from build123d import *

# Parameters (mm, degrees)
F1_DEPTH = 8.1
F3_DEPTH = 0.7
F5_DEPTH = 4.1
F6_DEPTH = 2.7


with BuildPart() as f1:
    # F0 (on Top) → F1 (new body)
    with BuildSketch(Plane.XY):
        Polygon((-9.85, -9.65), (9.85, -9.65), (9.85, 5.25), (13.5, 5.25), (13.5, 5.95), (9.85, 5.95), (9.85, 9.65), (-9.85, 9.65), (-9.85, 5.95), (-13.5, 5.95), (-13.5, 5.25), (-9.85, 5.25), align=None)
    extrude(amount=F1_DEPTH)

    # F2 (on face) → F3 (cut, through all)
    with BuildSketch(Plane(origin=(0, 5.95, 0), x_dir=(-1, 0, 0), z_dir=(0, 1, 0))):
        with BuildLine():
            ThreePointArc((-11.65, 0), (-13.015604, 1.823736), (-13.5, 4.05))
            Line((-13.5, 4.05), (-13.5, 0))
            Line((-13.5, 0), (-11.65, 0))
        make_face()
        with BuildLine():
            ThreePointArc((-13.5, 4.05), (-13.015604, 6.276264), (-11.65, 8.1))
            Line((-11.65, 8.1), (-13.5, 8.1))
            Line((-13.5, 8.1), (-13.5, 4.05))
        make_face()
        with BuildLine():
            Line((13.5, 8.1), (11.65, 8.1))
            ThreePointArc((11.65, 8.1), (13.015604, 6.276264), (13.5, 4.05))
            Line((13.5, 4.05), (13.5, 8.1))
        make_face()
        with BuildLine():
            Line((13.5, 0), (13.5, 4.05))
            ThreePointArc((13.5, 4.05), (13.015604, 1.823736), (11.65, 0))
            Line((11.65, 0), (13.5, 0))
        make_face()
    extrude(amount=-F3_DEPTH, mode=Mode.SUBTRACT)

    # F4 (on face) → F5 (join)
    with BuildSketch(Plane(origin=(0, 9.65, 0), x_dir=(-1, 0, 0), z_dir=(0, 1, 0))):
        with BuildLine():
            ThreePointArc((5.8, 8.1), (3.82183, 7.584027), (2.347701, 6.167577))
            ThreePointArc((2.347701, 6.167577), (1.75, 4.05), (2.347701, 1.932423))
            ThreePointArc((2.347701, 1.932423), (3.82183, 0.515973), (5.8, 0))
            ThreePointArc((5.8, 0), (8.663782, 1.186218), (9.85, 4.05))
            ThreePointArc((9.85, 4.05), (8.663782, 6.913782), (5.8, 8.1))
        make_face()
    extrude(amount=F5_DEPTH)

    # F4 (on face) → F6 (join)
    with BuildSketch(Plane(origin=(0, 9.65, 0), x_dir=(-1, 0, 0), z_dir=(0, 1, 0))):
        with BuildLine():
            ThreePointArc((2.347701, 1.932423), (1.75, 4.05), (2.347701, 6.167577))
            ThreePointArc((2.347701, 6.167577), (-0.85, 4.05), (2.347701, 1.932423))
        make_face()
    extrude(amount=F6_DEPTH)


solid = f1.part
For this review, take the finished solid that the model builds, in its own axes (mm). A direction names the side the tool comes from. Round coordinates to 2 decimals unless told otherwise and drop trailing zeros. Order: outer loops, then holes, each group sorted by start corner. A loop starts at its lowest first (then second) coordinate and runs counter-clockwise, first axis right, second up. Notation, with made-up numbers: M -29.5,42.25 L 12.5,42.25 A13 ccw 12.5,67.25 Z; hole C 87.25,-33.5 d1. An arc over 180 degrees is marked long. Use a Markdown table: item, result. Add a question column.
Item 1: Insertion check: pin 1 (4 mm diameter, centred on y = 8, z = 4.5, fed in from -X); pin 2 (2.5 mm diameter, centred on x = 0, z = 3, fed in from +Y); pin 3 (1.8 mm diameter, centred on x = 11, z = 4, fed in from -Y). Each pin has a flat end and moves straight along its axis. Give the tip position at first contact, or say it passes through.
Item 2: Add section C-C, the plane z = 5. Give the boundary of the cut face in (x, y).
Item 3: To check wall thickness, follow line 1 along X through (y, z) = (1.5, 6.75); line 2 along Y through (x, z) = (3.25, 6.25); line 3 along Y through (x, z) = (-12, 6.75). State the ranges of each line that lie inside material, in increasing order.
Item 4: Tool access review of faces 1 (the flat face through (11, 5.25, 4)), 2 (the flat face through (-9, 9.65, 7)), 3 (the flat face through (9.85, 8, 4)), 4 (the flat face through (-11, 5.25, 4)): name each direction out of +Z, -Z, +X, -X, +Y, -Y from which nothing blocks a thin tool from reaching the whole face with its end or side.
Item 5: Add section D-D, the plane y = -5.75. Give the boundary of the cut face in (x, z), then the cut area to 3 significant figures.
Item 6: Add section B-B, the plane y = 11.25. Give the boundary of the cut face in (x, z), then the cut area to 3 significant figures.
Item 7: Add section A-A, the plane x = -1.45. Give the boundary of the cut face in (y, z).
Item 8: Mouldability with a two-part tool opening along X and no side actions: class faces 5 (the cylindrical face through (0.85, 10.98, 4.11)), 6 (the flat face through (9.85, -2, 4)), 7 (the flat face through (-11, 5.95, 4)) as released by +X, released by -X, zero draft, split by the parting line, or undercut.
Geometry results:
| question | item | result |
|---|---|---|
| 1 | pin 1 | stops at x = -9.85 |
| 1 | pin 2 | stops at y = 12.35 |
| 1 | pin 3 | stops at y = 5.25 |
| 2 | outline | M -13.42,5.25 L -9.85,5.25 L -9.85,-9.65 L 9.85,-9.65 L 9.85,5.25 L 13.42,5.25 L 13.42,5.95 L 9.85,5.95 L 9.85,9.65 L 0.64,9.65 L 0.64,12.35 L -1.86,12.35 L -1.86,13.75 L -9.74,13.75 L -9.74,9.65 L -9.85,9.65 L -9.85,5.95 L -13.42,5.95 Z |
| 3 | line 1 | x = -9.85 to 9.85 |
| 3 | line 2 | y = -9.65 to 9.65 |
| 3 | line 3 | y = 5.25 to 5.95 |
| 4 | face 1 | +Z, -Z, +X, -Y |
| 4 | face 2 | +Z, -X, +Y |
| 4 | face 3 | +Z, -Z, +X, +Y |
| 4 | face 4 | +Z, -Z, -X, -Y |
| 5 | outline | M -9.85,0 L 9.85,0 L 9.85,8.1 L -9.85,8.1 Z |
| 5 | area | 160 mm² |
| 6 | outline | M -9.85,4.05 A4.05 ccw -5.8,0 A4.05 ccw -2.35,1.93 A2.3 ccw long -2.35,6.17 A4.05 ccw -5.8,8.1 A4.05 ccw Z |
| 6 | area | 62.1 mm² |
| 7 | outline | M -9.65,0 L 9.65,0 L 9.65,1.75 L 12.35,1.75 L 12.35,6.35 L 9.65,6.35 L 9.65,8.1 L -9.65,8.1 Z |
| 8 | face 5 | undercut |
| 8 | face 6 | released by +X |
| 8 | face 7 | zero draft |
